Work out the finished part from the listing and answer in its coordinate system (mm). Face numbers are marked on the shaded views. A direction names the side the tool comes from. Round coordinates to 2 decimals unless told otherwise and drop trailing zeros. Loops run counter-clockwise (first coordinate to the right, second up) from the corner with the lowest first, then second, coordinate; pieces in that order, holes last. Notation, with made-up numbers: (48.5, 61.25) -> (62.5, 61.25) arc R24 cw to (62.5, 92.25) -> close; hole circle Ø7 at (49, 26.25). An arc over 180 degrees is marked (long way). Use one line per item in the form item = value.
```python
from build123d import *

# Parameters (mm, degrees)
SKETCH1_W           = 58.7375
SKETCH1_H           = 93.6625
BACK_DEPTH          = 2.38125
SKETCH2_W           = 58.7375
SKETCH2_H           = 93.6625
SKETCH2_W_2         = 53.975
SKETCH2_H_2         = 88.9
SIDES_DEPTH         = 80.16875
SKETCH6_R           = 1.35255
BOSS_EXTRUDE6_DEPTH = 25.4
SKETCH5_W           = 22.225
SKETCH5_H           = 28.575
BOSS_EXTRUDE5_DEPTH = 2.38125
FILLET4_R           = 2.38125
FILLET5_R           = 0.79375


with BuildPart() as part:
    # Sketch1 → Back (new body)
    with BuildSketch(Plane.XY):
        Rectangle(SKETCH1_W, SKETCH1_H)
    extrude(amount=BACK_DEPTH)

    # Sketch2 → Sides (add)
    with BuildSketch(Plane.XY.offset(2.38125)):
        Rectangle(SKETCH2_W, SKETCH2_H)
        Rectangle(SKETCH2_W_2, SKETCH2_H_2, mode=Mode.SUBTRACT)
    extrude(amount=SIDES_DEPTH)

    # Sketch6 → Boss-Extrude6 (add)
    # profile 1 of 2: a face of its own
    with BuildSketch(Plane.XY.offset(82.55)):
        with BuildLine():
            Line((-3.7338, 40.379264529), (-3.7338, 44.45))
            Line((-3.7338, 44.45), (3.7338, 44.45))
            Line((3.7338, 44.45), (3.7338, 40.379264529))
            ThreePointArc((3.7338, 40.379264529), (0, 36.645464529), (-3.7338, 40.379264529))
        make_face()
        with Locations((0, 40.379264529)):
            Circle(SKETCH6_R, mode=Mode.SUBTRACT)
    # profile 2 of 2: a face of its own
    with BuildSketch(Plane.XY.offset(82.55)):
        with BuildLine():
            Line((-3.7338, -40.48125), (-3.7338, -44.45))
            Line((-3.7338, -44.45), (3.7338, -44.45))
            Line((3.7338, -44.45), (3.7338, -40.48125))
            ThreePointArc((3.7338, -40.48125), (0, -36.74745), (-3.7338, -40.48125))
        make_face()
        with Locations((0, -40.48125)):
            Circle(SKETCH6_R, mode=Mode.SUBTRACT)
    extrude(amount=-BOSS_EXTRUDE6_DEPTH)

    # Sketch5 → Boss-Extrude5 (add)
    with BuildSketch(Plane(origin=(29.36875, 0, 0), x_dir=(0, 0, -1), z_dir=(1, 0, 0))):
        with Locations((-58.7375, 61.11875)):
            Rectangle(SKETCH5_W, SKETCH5_H)
        with Locations((-58.7375, -61.11875)):
            Rectangle(SKETCH5_W, SKETCH5_H)
    extrude(amount=-BOSS_EXTRUDE5_DEPTH)

    # Fillet4
    fillet4_edges = [part.edges().sort_by_distance(p)[0] for p in [
        (26.9875, 0, 2.38125),
        (0, -44.45, 2.38125),
        (-26.9875, 0, 2.38125),
        (0, 44.45, 2.38125),
        (0, 46.83125, 0),
        (-29.36875, 0, 0),
        (0, -46.83125, 0),
        (29.36875, 0, 0),
        (-26.9875, -44.45, 42.465625),
        (-26.9875, 44.45, 42.465625),
        (26.9875, 44.45, 42.465625),
        (26.9875, -44.45, 42.465625),
        (29.36875, 46.83125, 23.8125),
        (29.36875, -46.83125, 23.8125),
        (29.36875, -46.83125, 76.2),
        (29.36875, 46.83125, 76.2),
        (-29.36875, -46.83125, 41.275),
        (-29.36875, 46.83125, 41.275),
    ]]
    fillet(fillet4_edges, radius=FILLET4_R)

    # Fillet5
    fillet5_edges = [part.edges().sort_by_distance(p)[0] for p in [
        (-26.290048023, -43.752548023, 82.55),
        (-26.290048023, 43.752548023, 82.55),
        (26.290048023, 43.752548023, 82.55),
        (26.290048023, -43.752548023, 82.55),
        (-14.170025, 44.45, 82.55),
        (0, 44.45, 57.15),
        (-3.7338, 44.45, 69.85),
        (3.7338, 44.45, 69.85),
        (0, 36.645464529, 82.55),
        (3.7338, 42.414632265, 82.55),
        (-3.7338, 42.414632265, 82.55),
        (14.170025, -44.45, 82.55),
        (-3.7338, -44.45, 69.85),
        (0, -36.74745, 82.55),
        (-3.7338, -42.465625, 82.55),
        (3.7338, -42.465625, 82.55),
        (26.9875, 0, 82.55),
        (-14.170025, -44.45, 82.55),
        (-26.9875, 0, 82.55),
        (14.170025, 44.45, 82.55),
    ]]
    fillet(fillet5_edges, radius=FILLET5_R)


solid = part.part
```
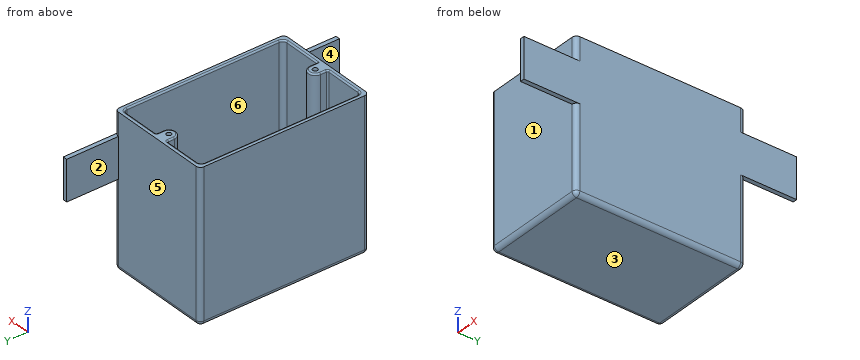
(1) Find section A-A, the plane z = 72.5. State how many separate pieces and enclosed holes the cut face has, then the cut area to 3 significant figures.
Completed:
separate_pieces = 1
enclosed_holes = 3
area = 796 mm2
(2) Find section C-C, the plane z = 44. Write down the section's boundary in (x, y).
Completed:
outline = (-29.37, -44.45) arc R2.38 ccw to (-26.99, -46.83) -> (26.99, -46.83) arc R2.38 ccw to (29.37, -44.45) -> (29.37, 44.45) arc R2.38 ccw to (26.99, 46.83) -> (-26.99, 46.83) arc R2.38 ccw to (-29.37, 44.45) -> close; hole (-26.99, -42.07) arc R2.38 ccw to (-24.61, -44.45) -> (24.61, -44.45) arc R2.38 ccw to (26.99, -42.07) -> (26.99, 42.07) arc R2.38 ccw to (24.61, 44.45) -> (-24.61, 44.45) arc R2.38 ccw to (-26.99, 42.07) -> close
(3) Given P1, Ø2.5, axis at x = 28.5, y = -60.5, coming from the +Z side; P2, Ø15, axis at x = 3, z = 40.5, coming from the -Y side; P3, Ø4, axis at x = -17.5, y = -30.5, coming from the +Z side, each flat-ended and moving along its own axis, determine where each tip first touches the part or whether it passes through.
Completed:
P1 = 69.85
P2 = -46.83
P3 = 2.38
(4) For a pull along Y with two mould halves and no side action, classify the marked faces 4, 5 and 6 as +Y half, -Y half, draft (parallel to the pull), parting line (faces both ways), or undercut.
Completed:
face_4 = draft
face_5 = +Y half
face_6 = undercut
(5) Consider L1, parallel to Y at x = 0, z = 63; L2, parallel to X at y = 17.5, z = 77; L3, parallel to Z at x = 0, y = -23. Determine where each line is inside the solid, lowest interval first.
Completed:
L1 = -46.83 to -41.83, -39.13 to -36.75, 36.65 to 39.03, 41.73 to 46.83
L2 = -29.37 to -26.99, 26.99 to 29.37
L3 = 0 to 2.38
(6) Find section B-B, the plane x = -9.5. Write down the section's boundary in (y, z), then the cut area to 3 significant figures.
Completed:
outline = (-46.83, 2.38) arc R2.38 ccw to (-44.45, 0) -> (44.45, 0) arc R2.38 ccw to (46.83, 2.38) -> (46.83, 82.55) -> (45.24, 82.55) arc R0.79 ccw to (44.45, 81.76) -> (44.45, 4.76) arc R2.38 cw to (42.07, 2.38) -> (-42.07, 2.38) arc R2.38 cw to (-44.45, 4.76) -> (-44.45, 81.76) arc R0.79 ccw to (-45.24, 82.55) -> (-46.83, 82.55) -> close
area = 605 mm2
(7) For the marked faces 1, 2 and 3, determine the directions among +Z, -Z, +X, -X, +Y, -Y from which every point of the face is accessible in a straight line to the end or side of a thin tool.
Completed:
face_1 = +Z, -Z, -X, -Y
face_2 = +Z, -Z, -X, +Y
face_3 = -Z, +X, -X, +Y, -Y
(8) Find section D-D, the plane y = -8. Write down the section's boundary in (x, z), then the cut area to 3 significant figures.
Completed:
outline = (-29.37, 2.38) arc R2.38 ccw to (-26.99, 0) -> (26.99, 0) arc R2.38 ccw to (29.37, 2.38) -> (29.37, 82.55) -> (27.78, 82.55) arc R0.79 ccw to (26.99, 81.76) -> (26.99, 4.76) arc R2.38 cw to (24.61, 2.38) -> (-24.61, 2.38) arc R2.38 cw to (-26.99, 4.76) -> (-26.99, 81.76) arc R0.79 ccw to (-27.78, 82.55) -> (-29.37, 82.55) -> close
area = 521 mm2
